```python
from build123d import *

# Parameters (mm, degrees)
F1_DEPTH = 20
F2_DEPTH = 20
F3_DEPTH = 10


with BuildPart() as f1:
    # F0 (on Front) → F1 (new body, symmetric)
    with BuildSketch(Plane.XZ):
        Polygon((0, 60), (0, 0), (30, 0), (30, 50), (20, 60), align=None)
    extrude(amount=F1_DEPTH, both=True)

    # F0 (on Front) → F2 (join, symmetric)
    with BuildSketch(Plane.XZ):
        Polygon((30, 50), (30, 0), (60, 0), (60, 20), align=None)
    extrude(amount=F2_DEPTH, both=True)

    # F0 (on Front) → F3 (cut, symmetric)
    with BuildSketch(Plane.XZ):
        Polygon((30, 50), (30, 0), (60, 0), (60, 20), align=None)
    extrude(amount=F3_DEPTH, both=True, mode=Mode.SUBTRACT)


solid = f1.part
```
Input: part model. Units: mm. Frame: model coordinates. A direction names the side the tool comes from. Round coordinates to 2 decimals unless told otherwise and drop trailing zeros. Write each loop counter-clockwise with the first axis right and the second up, starting at its lowest first coordinate (ties: lowest second). Pieces come first, ordered by that corner, then holes. Notation, with made-up numbers: (80.25, -27) - (92.25, -27) arc R19 cw to (92.25, -15) - close; hole circle Ø6 at (-4.5, 7). An arc over 180 degrees is marked (long way). Write item = value, one per line.
(1) Material intervals for probe 1 along Y at (x, z) = (36.5, 11.5); probe 2 along X at (y, z) = (1.5, 16); probe 3 along Z at (x, y) = (24, 15.5), sorted ascending.
Geometry check:
probe_1 = -20 to -10, 10 to 20
probe_2 = 0 to 30
probe_3 = 0 to 56
(2) Section query B-B on z = 29. Output: boundary loops of the cut face in (x, y), then the cut area to 3 significant figures.
Geometry check:
outline = (0, -20) - (51, -20) - (51, -10) - (30, -10) - (30, 10) - (51, 10) - (51, 20) - (0, 20) - close
area = 1,620 mm^2
(3) Section query A-A on x = 31. Output: boundary loops of the cut face in (y, z).
Geometry check:
outline = (-20, 0) - (-10, 0) - (-10, 49) - (-20, 49) - close; (10, 0) - (20, 0) - (20, 49) - (10, 49) - close
(4) Section query C-C on x = 49. Output: boundary loops of the cut face in (y, z).
Geometry check:
outline = (-20, 0) - (-10, 0) - (-10, 31) - (-20, 31) - close; (10, 0) - (20, 0) - (20, 31) - (10, 31) - close
(5) Section query D-D on y = 15.5. Output: boundary loops of the cut face in (x, z).
Geometry check:
outline = (0, 0) - (60, 0) - (60, 20) - (20, 60) - (0, 60) - close
(6) Access query for faces 1 (the flat face through (41, -10, 20)), 2 (the flat face through (0, 0, 30)). Directions: +Z, -Z, +X, -X, +Y, -Y. A direction counts if a zero-diameter tool reaches every point of the face in a straight line with its end or side. Return the directions, or none.
Geometry check:
face_1 = +Z, -Z, +X
face_2 = +Z, -Z, -X, +Y, -Y
(7) Pull-direction query (Y, two-part tool) for faces 3 (the flat face through (41, 10, 20)), 4 (the flat face through (60, -15, 10)), 5 (the flat face through (23, 20, 24)), 6 (the flat face through (30, 0, 25)); classes: +Y half, -Y half, draft (parallel to the pull), parting line (faces both ways), or undercut.
Geometry check:
face_3 = undercut
face_4 = draft
face_5 = +Y half
face_6 = undercut
